Can you work these out from the model? Positions are in its coordinate system, mm. A direction names the side the tool comes from. Round coordinates to 2 decimals unless told otherwise and drop trailing zeros. Write each loop counter-clockwise with the first axis right and the second up, starting at its lowest first coordinate (ties: lowest second). Pieces come first, ordered by that corner, then holes. Notation, with made-up numbers: M -25.5,70.25 L -19.5,70.25 A12 cw -19.5,84.25 Z; hole C 74.25,37 d8. An arc over 180 degrees is marked long. Answer in a Markdown table with one row per item. Add a question column.
(1) If I drill on probe 1 along Y at (x, z) = (0, -0.6); probe 2 along X at (y, z) = (-13, -0.9); probe 3 along X at (y, z) = (2, -0.05), over which ranges is the centre line in solid material (lowest first)?
(2) For faces 1 (the face through (-0.325, 11.036, -0.493)), 2 (the face through (0, 0, -1.5)), which set-ups out of +Z, -Z, +X, -X, +Y, -Y let a thin tool reach every point of the face, with its end or its side?
(3) Suppose I cut it at D-D, the plane x = 6. Write out the boundary of the cut face in (y, z).
(4) If we mould it in two halves opening along Y, with no side actions, what happens to faces 3 (the face through (0, 13, -1)), 4 (the face through (0, 0, 0)), 5 (the face through (-3.47, -15.62, -0.74))? For each: released by +Y, released by -Y, zero draft, split by the parting line, or undercut.
(5) Suppose I cut it at C-C, the plane y = 12.5. Write out the boundary of the cut face in (x, z), then the cut area to 3 significant figures.
(6) I'm going to push a flat-ended pin straight in: pin 1 (0.9 mm diameter, centred on x = 0, y = -13, fed in from +Z). Where does the tip first touch, or does it pass through?
(7) Suppose I cut it at B-B, the plane z = -0.6. Write out the boundary of the cut face in (x, y), then the cut area to 3 significant figures.
(8) Suppose I cut it at A-A, the plane x = 0. Write out the boundary of the cut face in (y, z), then the cut area to 3 significant figures.
from build123d import *

# Parameters (mm, degrees)
SCHIZZO1_R                   = 16
ESTRUSIONE_ESTRUSIONE1_DEPTH = 1.5
SCHIZZO7_R                   = 1.5
TAGLIO_ESTRUSIONE1_DEPTH     = 1
RIPETIZIONECIRCOLARE1_COUNT  = 4


with BuildPart() as part:
    # Schizzo1 → Estrusione-Estrusione1 (new body)
    with BuildSketch(Plane.XY):
        Circle(SCHIZZO1_R)
    extrude(amount=-ESTRUSIONE_ESTRUSIONE1_DEPTH)

    # Schizzo7 → Taglio-Estrusione1 (cut)
    with BuildSketch(Plane.XY):
        with Locations((0, 12.5)):
            Circle(SCHIZZO7_R)
    taglio_estrusione1 = extrude(amount=-TAGLIO_ESTRUSIONE1_DEPTH, mode=Mode.SUBTRACT)

    # RipetizioneCircolare1: Taglio-Estrusione1 ×4 about axis
    ripetizionecircolare1_axis = Axis((0, -0.110837438, 0), (0, 0, 1))
    for i in range(1, RIPETIZIONECIRCOLARE1_COUNT):
        add(taglio_estrusione1.rotate(ripetizionecircolare1_axis, i * 360 / RIPETIZIONECIRCOLARE1_COUNT), mode=Mode.SUBTRACT)


solid = part.part
Calculated:
| question | item | result |
|---|---|---|
| 1 | probe 1 | -16 to -14.22, -11.22 to 11, 14 to 16 |
| 1 | probe 2 | -9.33 to -1.47, 1.47 to 9.33 |
| 1 | probe 3 | -15.87 to 15.87 |
| 2 | face 1 | +Z |
| 2 | face 2 | -Z, +X, -X, +Y, -Y |
| 3 | outline | M -14.83,-1.5 L 14.83,-1.5 L 14.83,0 L -14.83,0 Z |
| 4 | face 3 | undercut |
| 4 | face 4 | zero draft |
| 4 | face 5 | split by the parting line |
| 5 | outline | M -9.99,-1.5 L 9.99,-1.5 L 9.99,0 L 1.5,0 L 1.5,-1 L -1.5,-1 L -1.5,0 L -9.99,0 Z |
| 5 | area | 27.0 mm² |
| 6 | pin 1 | z = -1 |
| 7 | outline | C 0,0 d32; hole C -12.61,-0.11 d3; hole C 0,-12.72 d3; hole C 0,12.5 d3; hole C 12.61,-0.11 d3 |
| 7 | area | 776 mm² |
| 8 | outline | M -16,-1.5 L 16,-1.5 L 16,0 L 14,0 L 14,-1 L 11,-1 L 11,0 L -11.22,0 L -11.22,-1 L -14.22,-1 L -14.22,0 L -16,0 Z |
| 8 | area | 42.0 mm² |
